```python
from build123d import *

# Parameters (mm, degrees)
SKETCH1_W           = 240
SKETCH1_H           = 151
BOSS_EXTRUDE1_DEPTH = 5
SKETCH2_W           = 27
SKETCH2_H           = 45
CUT_EXTRUDE1_DEPTH  = 10
CUT_EXTRUDE10_DEPTH = 5
SKETCH15_R          = 2.5
CUT_EXTRUDE11_DEPTH = 10
SKETCH17_R          = 2
SKETCH17_W          = 30
SKETCH17_H          = 5.2
CUT_EXTRUDE13_DEPTH = 10
SKETCH20_R          = 2
CUT_EXTRUDE15_DEPTH = 5
SKETCH23_R          = 2
CUT_EXTRUDE16_DEPTH = 5
SKETCH24_W          = 30.2
SKETCH24_H          = 5.2
CUT_EXTRUDE17_DEPTH = 5
SKETCH27_R          = 1.5
CUT_EXTRUDE20_DEPTH = 10
SKETCH28_R          = 2
CUT_EXTRUDE21_DEPTH = 10
SKETCH31_R          = 2
CUT_EXTRUDE24_DEPTH = 10
SKETCH32_R          = 2
CUT_EXTRUDE25_DEPTH = 10
SKETCH34_W          = 40
SKETCH34_H          = 42
CUT_EXTRUDE26_DEPTH = 10
CUT_EXTRUDE27_DEPTH = 10
CUT_EXTRUDE28_DEPTH = 10
SKETCH37_W          = 5.2
SKETCH37_H          = 20.2
CUT_EXTRUDE29_DEPTH = 10
SKETCH38_W          = 20.2
SKETCH38_H          = 5.02
CUT_EXTRUDE30_DEPTH = 5
SKETCH39_R          = 2
CUT_EXTRUDE31_DEPTH = 5
SKETCH40_R          = 4
SKETCH40_R_2        = 2
BOSS_EXTRUDE6_DEPTH = 5
FILLET1_R           = 3
SKETCH41_R          = 2
CUT_EXTRUDE32_DEPTH = 5
SKETCH42_R          = 4
SKETCH42_R_2        = 2
BOSS_EXTRUDE7_DEPTH = 5
SKETCH43_W          = 5
SKETCH43_H          = 30
BOSS_EXTRUDE8_DEPTH = 5
FILLET2_R           = 3


with BuildPart() as part:
    # Sketch1 → Boss-Extrude1 (new body)
    with BuildSketch(Plane.XY):
        Rectangle(SKETCH1_W, SKETCH1_H)
    extrude(amount=BOSS_EXTRUDE1_DEPTH)

    # Sketch2 → Cut-Extrude1 (cut)
    with BuildSketch(Plane(origin=(0, 0, 0), x_dir=(-1, 0, 0), z_dir=(0, 0, -1))):
        with Locations((23.5, -1.5)):
            Rectangle(SKETCH2_W, SKETCH2_H)
        with Locations((-23.5, -1.5)):
            Rectangle(SKETCH2_W, SKETCH2_H)
    extrude(amount=-CUT_EXTRUDE1_DEPTH, mode=Mode.SUBTRACT)

    # Sketch14 → Cut-Extrude10 (cut)
    with BuildSketch(Plane(origin=(0, 0, 0), x_dir=(-1, 0, 0), z_dir=(0, 0, -1))):
        with BuildLine():
            Line((-56.3, 15.46), (-52.3, 15.46))
            ThreePointArc((-52.3, 15.46), (-50.3, 13.46), (-52.3, 11.46))
            Line((-52.3, 11.46), (-56.3, 11.46))
            ThreePointArc((-56.3, 11.46), (-58.3, 13.46), (-56.3, 15.46))
        make_face()
        with BuildLine():
            Line((-80.3, 15.46), (-76.3, 15.46))
            ThreePointArc((-76.3, 15.46), (-74.3, 13.46), (-76.3, 11.46))
            Line((-76.3, 11.46), (-80.3, 11.46))
            ThreePointArc((-80.3, 11.46), (-82.3, 13.46), (-80.3, 15.46))
        make_face()
        with BuildLine():
            Line((-80.3, -14.54), (-76.3, -14.54))
            ThreePointArc((-76.3, -14.54), (-74.3, -16.54), (-76.3, -18.54))
            Line((-76.3, -18.54), (-80.3, -18.54))
            ThreePointArc((-80.3, -18.54), (-82.3, -16.54), (-80.3, -14.54))
        make_face()
        with BuildLine():
            Line((-56.3, -14.54), (-52.3, -14.54))
            ThreePointArc((-52.3, -14.54), (-50.3, -16.54), (-52.3, -18.54))
            Line((-52.3, -18.54), (-56.3, -18.54))
            ThreePointArc((-56.3, -18.54), (-58.3, -16.54), (-56.3, -14.54))
        make_face()
        with BuildLine():
            Line((56.3, -14.54), (52.3, -14.54))
            ThreePointArc((52.3, -14.54), (50.3, -16.54), (52.3, -18.54))
            Line((52.3, -18.54), (56.3, -18.54))
            ThreePointArc((56.3, -18.54), (58.3, -16.54), (56.3, -14.54))
        make_face()
        with BuildLine():
            Line((80.3, -14.54), (76.3, -14.54))
            ThreePointArc((76.3, -14.54), (74.3, -16.54), (76.3, -18.54))
            Line((76.3, -18.54), (80.3, -18.54))
            ThreePointArc((80.3, -18.54), (82.3, -16.54), (80.3, -14.54))
        make_face()
        with BuildLine():
            Line((80.3, 15.46), (76.3, 15.46))
            ThreePointArc((76.3, 15.46), (74.3, 13.46), (76.3, 11.46))
            Line((76.3, 11.46), (80.3, 11.46))
            ThreePointArc((80.3, 11.46), (82.3, 13.46), (80.3, 15.46))
        make_face()
        with BuildLine():
            Line((56.3, 15.46), (52.3, 15.46))
            ThreePointArc((52.3, 15.46), (50.3, 13.46), (52.3, 11.46))
            Line((52.3, 11.46), (56.3, 11.46))
            ThreePointArc((56.3, 11.46), (58.3, 13.46), (56.3, 15.46))
        make_face()
    extrude(amount=-CUT_EXTRUDE10_DEPTH, mode=Mode.SUBTRACT)

    # Sketch15 → Cut-Extrude11 (cut)
    with BuildSketch(Plane(origin=(0, 0, 0), x_dir=(-1, 0, 0), z_dir=(0, 0, -1))):
        with Locations((-102.2, -27)):
            Circle(SKETCH15_R)
        with Locations((-102.2, 24)):
            Circle(SKETCH15_R)
        with Locations((102.2, 24)):
            Circle(SKETCH15_R)
        with Locations((102.2, -27)):
            Circle(SKETCH15_R)
    extrude(amount=-CUT_EXTRUDE11_DEPTH, mode=Mode.SUBTRACT)

    # Sketch17 → Cut-Extrude13 (cut)
    with BuildSketch(Plane(origin=(0, 0, 0), x_dir=(-1, 0, 0), z_dir=(0, 0, -1))):
        with Locations((-29.9, -39.1)):
            Circle(SKETCH17_R)
        with Locations((29.9, -39.1)):
            Circle(SKETCH17_R)
        with Locations((-29.9, 36.1)):
            Circle(SKETCH17_R)
        with Locations((29.9, 36.1)):
            Circle(SKETCH17_R)
        with Locations((0, 36.1)):
            Rectangle(SKETCH17_W, SKETCH17_H)
        with Locations((0, -39.1)):
            Rectangle(SKETCH17_W, SKETCH17_H)
    extrude(amount=-CUT_EXTRUDE13_DEPTH, mode=Mode.SUBTRACT)

    # Sketch20 → Cut-Extrude15 (cut)
    with BuildSketch(Plane(origin=(0, 0, 0), x_dir=(-1, 0, 0), z_dir=(0, 0, -1))):
        with Locations((43.2, 67)):
            Circle(SKETCH20_R)
        with Locations((-43.2, 67)):
            Circle(SKETCH20_R)
    extrude(amount=-CUT_EXTRUDE15_DEPTH, mode=Mode.SUBTRACT)

    # Sketch23 → Cut-Extrude16 (cut)
    with BuildSketch(Plane(origin=(0, 0, 0), x_dir=(-1, 0, 0), z_dir=(0, 0, -1))):
        with Locations((42.8, -54)):
            Circle(SKETCH23_R)
        with Locations((-42.8, -54)):
            Circle(SKETCH23_R)
    extrude(amount=-CUT_EXTRUDE16_DEPTH, mode=Mode.SUBTRACT)

    # Sketch24 → Cut-Extrude17 (cut)
    with BuildSketch(Plane(origin=(0, 0, 0), x_dir=(-1, 0, 0), z_dir=(0, 0, -1))):
        with Locations((0, -54.1)):
            Rectangle(SKETCH24_W, SKETCH24_H)
    extrude(amount=-CUT_EXTRUDE17_DEPTH, mode=Mode.SUBTRACT)

    # Sketch27 → Cut-Extrude20 (cut)
    with BuildSketch(Plane(origin=(0, 0, 0), x_dir=(-1, 0, 0), z_dir=(0, 0, -1))):
        with Locations((-25, 25)):
            Circle(SKETCH27_R)
        with Locations((0, 25)):
            Circle(SKETCH27_R)
        with Locations((25, 25)):
            Circle(SKETCH27_R)
    extrude(amount=-CUT_EXTRUDE20_DEPTH, mode=Mode.SUBTRACT)

    # Sketch28 → Cut-Extrude21 (cut)
    with BuildSketch(Plane.XY.offset(5)):
        with Locations((112, -52.5)):
            Circle(SKETCH28_R)
        with Locations((65, -52.5)):
            Circle(SKETCH28_R)
        with Locations((-65, -52.5)):
            Circle(SKETCH28_R)
        with Locations((-112, -52.5)):
            Circle(SKETCH28_R)
    extrude(amount=-CUT_EXTRUDE21_DEPTH, mode=Mode.SUBTRACT)

    # Sketch31 → Cut-Extrude24 (cut)
    with BuildSketch(Plane(origin=(0, 0, 0), x_dir=(-1, 0, 0), z_dir=(0, 0, -1))):
        with Locations((72.345744872, -69.339745962)):
            Circle(SKETCH31_R)
        with Locations((-72.345744872, -69.339745962)):
            Circle(SKETCH31_R)
    extrude(amount=-CUT_EXTRUDE24_DEPTH, mode=Mode.SUBTRACT)

    # Sketch32 → Cut-Extrude25 (cut)
    with BuildSketch(Plane(origin=(0, 0, 0), x_dir=(-1, 0, 0), z_dir=(0, 0, -1))):
        with Locations((52.005844325, -34.1100048)):
            Circle(SKETCH32_R)
        with Locations((-52.005844325, -34.1100048)):
            Circle(SKETCH32_R)
    extrude(amount=-CUT_EXTRUDE25_DEPTH, mode=Mode.SUBTRACT)

    # Sketch34 → Cut-Extrude26 (cut)
    with BuildSketch(Plane(origin=(0, 0, 0), x_dir=(-1, 0, 0), z_dir=(0, 0, -1))):
        with Locations((-100, 54.5)):
            Rectangle(SKETCH34_W, SKETCH34_H)
    extrude(amount=-CUT_EXTRUDE26_DEPTH, mode=Mode.SUBTRACT)

    # Sketch35 → Cut-Extrude27 (cut)
    with BuildSketch(Plane(origin=(0, 0, 0), x_dir=(-1, 0, 0), z_dir=(0, 0, -1))):
        with BuildLine():
            Line((-49.5, 32.5), (-69.5, 32.5))
            ThreePointArc((-69.5, 32.5), (-74.5, 37.5), (-69.5, 42.5))
            Line((-69.5, 42.5), (-49.5, 42.5))
            ThreePointArc((-49.5, 42.5), (-44.5, 37.5), (-49.5, 32.5))
        make_face()
    extrude(amount=-CUT_EXTRUDE27_DEPTH, mode=Mode.SUBTRACT)

    # Sketch36 → Cut-Extrude28 (cut)
    with BuildSketch(Plane(origin=(0, 0, 0), x_dir=(-1, 0, 0), z_dir=(0, 0, -1))):
        with BuildLine():
            Line((109, 35.5), (109, 55.5))
            ThreePointArc((109, 55.5), (112, 58.5), (115, 55.5))
            Line((115, 55.5), (115, 35.5))
            ThreePointArc((115, 35.5), (112, 32.5), (109, 35.5))
        make_face()
    extrude(amount=-CUT_EXTRUDE28_DEPTH, mode=Mode.SUBTRACT)

    # Sketch37 → Cut-Extrude29 (cut)
    with BuildSketch(Plane.XY.offset(5)):
        with Locations((34.6, 53.35)):
            Rectangle(SKETCH37_W, SKETCH37_H)
        with Locations((-34.6, 53.35)):
            Rectangle(SKETCH37_W, SKETCH37_H)
    extrude(amount=-CUT_EXTRUDE29_DEPTH, mode=Mode.SUBTRACT)

    # Sketch38 → Cut-Extrude30 (cut)
    with BuildSketch(Plane.XY.offset(5)):
        with Locations((-61.9, 21.51)):
            Rectangle(SKETCH38_W, SKETCH38_H)
    extrude(amount=-CUT_EXTRUDE30_DEPTH, mode=Mode.SUBTRACT)

    # Sketch39 → Cut-Extrude31 (cut)
    with BuildSketch(Plane(origin=(0, 0, 0), x_dir=(-1, 0, 0), z_dir=(0, 0, -1))):
        with Locations((107.8, 73)):
            Circle(SKETCH39_R)
    extrude(amount=-CUT_EXTRUDE31_DEPTH, mode=Mode.SUBTRACT)

    # Sketch40 → Boss-Extrude6 (add)
    with BuildSketch(Plane(origin=(0, 0, 0), x_dir=(-1, 0, 0), z_dir=(0, 0, -1))):
        with Locations((107.8, 73)):
            Circle(SKETCH40_R)
        with Locations((107.8, 73)):
            Circle(SKETCH40_R_2, mode=Mode.SUBTRACT)
    extrude(amount=-BOSS_EXTRUDE6_DEPTH)

    # Fillet1
    fillet1_edges = [part.edges().sort_by_distance(p)[0] for p in [
        (80, 33.5, 2.5),
    ]]
    fillet(fillet1_edges, radius=FILLET1_R)

    # Sketch41 → Cut-Extrude32 (cut)
    with BuildSketch(Plane(origin=(0, 0, 0), x_dir=(-1, 0, 0), z_dir=(0, 0, -1))):
        with Locations((39.8, -73)):
            Circle(SKETCH41_R)
        with Locations((-39.8, -73)):
            Circle(SKETCH41_R)
    extrude(amount=-CUT_EXTRUDE32_DEPTH, mode=Mode.SUBTRACT)

    # Sketch42 → Boss-Extrude7 (add)
    with BuildSketch(Plane(origin=(0, 0, 0), x_dir=(-1, 0, 0), z_dir=(0, 0, -1))):
        with Locations((-39.8, -73)):
            Circle(SKETCH42_R)
        with Locations((-39.8, -73)):
            Circle(SKETCH42_R_2, mode=Mode.SUBTRACT)
        with Locations((39.8, -73)):
            Circle(SKETCH42_R)
        with Locations((39.8, -73)):
            Circle(SKETCH42_R_2, mode=Mode.SUBTRACT)
    extrude(amount=-BOSS_EXTRUDE7_DEPTH)

    # Sketch43 → Boss-Extrude8 (add)
    with BuildSketch(Plane(origin=(0, 0, 0), x_dir=(-1, 0, 0), z_dir=(0, 0, -1))):
        with Locations((-122.5, 3.5)):
            Rectangle(SKETCH43_W, SKETCH43_H)
        with Locations((122.5, 24.5)):
            Rectangle(SKETCH43_W, SKETCH43_H)
    extrude(amount=-BOSS_EXTRUDE8_DEPTH)

    # Fillet2
    fillet2_edges = [part.edges().sort_by_distance(p)[0] for p in [
        (80, 75.5, 2.5),
    ]]
    fillet(fillet2_edges, radius=FILLET2_R)


solid = part.part
```
Build history of the part. All positions in model axes, mm. A direction names the side the tool comes from. Coordinates: 2 decimals unless noted, no trailing zeros. Order: outer loops, then holes, each group sorted by start corner. A loop starts at its lowest first (then second) coordinate and runs counter-clockwise, first axis right, second up. Notation, with made-up numbers: M 85.5,-17.5 L 96.5,-17.5 A18 ccw 96.5,0.5 Z; hole C 59.25,15 d8. An arc over 180 degrees is marked long. One line per question, with ' | ' between items. Start each with the question number.
1. Tool access for faces 4 (the face through (123, -11.5, 2)), 5 (the face through (-109, 45, 2)), 6 (the face through (-120, 57, 2)): list every direction of +Z, -Z, +X, -X, +Y, -Y with a clear straight run to the whole face (end or side of a thin tool).
2. Flat gauge pins, fed straight in: P1, Ø3, axis at x = -55, z = 3.5, coming from the -Y side; P2, Ø3.5, axis at x = -107.8, y = 73, coming from the -Z side; P3, Ø1, axis at y = 53, z = 2.5, coming from the -X side; P4, Ø3, axis at y = 52, z = 3.5, coming from the +X side. Where does each tip first touch, or does it go through?
3. Wall check: line 1 along X through (y, z) = (55, 4.15); line 2 along X through (y, z) = (-2, 2.15); line 3 along Y through (x, z) = (-102.2, 3.7). Give the ranges that are in metal, low to high. Write a range as [from, to].
4. Cut at B-B (y = -46.5). Write the cut outline in (x, z), plus the area to 3 significant figures.
5. Cut at A-A (y = -5.5). Write the cut outline in (x, z).
6. Cut at C-C (z = 1.9). Count the separate pieces of the cut face and the enclosed holes in it, plus the area to 3 significant figures.
7. Mould opens along Y. For faces 1 (the face through (81, -75.5, 2)), 2 (the face through (123, 18.5, 2)), 3 (the face through (35, 63.45, 3)) say: +Y half, -Y half, draft (parallel to the pull), parting line (faces both ways), or undercut.
The answers:
1) face 4: +Z, -Z, +X, -Y | face 5: +Z, -Z | face 6: +Z, -Z, -X, +Y
2) P1: stops at y = -75.5 | P2: passes through | P3: stops at x = -120 | P4: stops at x = 80
3) line 1: x = [-120, -115], [-109, -37.2], [-32, 32], [37.2, 80] | line 2: x = [-120, -37], [-10, 10], [37, 125] | line 3: y = [-75.5, -29.5], [-24.5, 21.5], [26.5, 75.5]
4) outline: M -120,0 L 120,0 L 120,5 L -120,5 Z | area: 1,200 mm2
5) outline: M -120,0 L -37,0 L -37,5 L -120,5 Z; M -10,0 L 10,0 L 10,5 L -10,5 Z; M 37,0 L 125,0 L 125,5 L 37,5 Z
6) separate pieces: 1 | enclosed holes: 44 | area: 30,700 mm2
7) face 1: -Y half | face 2: +Y half | face 3: undercut
